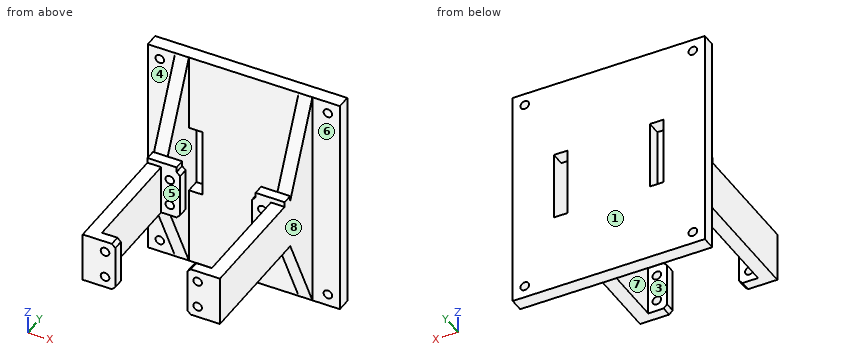
```python
from build123d import *

# Parameters (mm, degrees)
EXTRUDE_1_DEPTH      = 65
CUT_EXTRUDE_2_REACH  = 99.185
SKETCH_2_R           = 1.25
CUT_EXTRUDE_4_REACH  = 99.185
SKETCH_10_R          = 1.25
CUT_EXTRUDE_8_DEPTH  = 98.185389848
CUT_EXTRUDE_9_REACH  = 99.185
CUT_EXTRUDE_10_REACH = 99.185
SKETCH_25_W          = 8.5
SKETCH_25_H          = 3
EXTRUDE_2_DEPTH      = 1.5
SKETCH_26_W          = 8.5
SKETCH_26_H          = 3
EXTRUDE_3_DEPTH      = 1.5
CUT_EXTRUDE_11_REACH = 99.185


with BuildPart() as part:
    # 草图1 → 凸台-拉伸1 (new body)
    with BuildSketch(Plane.XY):
        Polygon((9.5, 3), (4, 3), (4, 35), (9.5, 35), (9.5, 38), (4, 38), (4, 50), (36, 50), (36, 38), (30.5, 38), (30.5, 35), (36, 35), (36, 3), (30.5, 3), (30.5, 0), (40, 0), (40, 50), (48, 50), (48, 54), (-8, 54), (-8, 50), (0, 50), (0, 0), (9.5, 0), align=None)
    extrude(amount=EXTRUDE_1_DEPTH)

    # 草图2 → 切除-拉伸2 (cut, up to next)
    with BuildSketch(Plane(origin=(0, 54, 0), x_dir=(1, 0, 0), z_dir=(0, 1, 0)), mode=Mode.PRIVATE) as cut_extrude_2_sk1:
        with Locations(Location((-4.5, -61.5, 0), (0, 0, 270))):
            Circle(SKETCH_2_R)
    cut_extrude_2_tool1 = extrude(cut_extrude_2_sk1.sketch, amount=-CUT_EXTRUDE_2_REACH, mode=Mode.PRIVATE) & part.part
    # 草图2 → 切除-拉伸2 (cut, up to next)
    with BuildSketch(Plane(origin=(0, 54, 0), x_dir=(1, 0, 0), z_dir=(0, 1, 0)), mode=Mode.PRIVATE) as cut_extrude_2_sk2:
        with Locations(Location((44.5, -61.5, 0), (0, 0, 270))):
            Circle(SKETCH_2_R)
    cut_extrude_2_tool2 = extrude(cut_extrude_2_sk2.sketch, amount=-CUT_EXTRUDE_2_REACH, mode=Mode.PRIVATE) & part.part
    # 草图2 → 切除-拉伸2 (cut, up to next)
    with BuildSketch(Plane(origin=(0, 54, 0), x_dir=(1, 0, 0), z_dir=(0, 1, 0)), mode=Mode.PRIVATE) as cut_extrude_2_sk3:
        with Locations(Location((44.5, -3.5, 0), (0, 0, 270))):
            Circle(SKETCH_2_R)
    cut_extrude_2_tool3 = extrude(cut_extrude_2_sk3.sketch, amount=-CUT_EXTRUDE_2_REACH, mode=Mode.PRIVATE) & part.part
    # 草图2 → 切除-拉伸2 (cut, up to next)
    with BuildSketch(Plane(origin=(0, 54, 0), x_dir=(1, 0, 0), z_dir=(0, 1, 0)), mode=Mode.PRIVATE) as cut_extrude_2_sk4:
        with Locations(Location((-4.5, -3.5, 0), (0, 0, 270))):
            Circle(SKETCH_2_R)
    cut_extrude_2_tool4 = extrude(cut_extrude_2_sk4.sketch, amount=-CUT_EXTRUDE_2_REACH, mode=Mode.PRIVATE) & part.part
    add(cut_extrude_2_tool1.solids().sort_by_distance((-4.5, 54, 61.5))[0], mode=Mode.SUBTRACT)
    add(cut_extrude_2_tool2.solids().sort_by_distance((44.5, 54, 61.5))[0], mode=Mode.SUBTRACT)
    add(cut_extrude_2_tool3.solids().sort_by_distance((44.5, 54, 3.5))[0], mode=Mode.SUBTRACT)
    add(cut_extrude_2_tool4.solids().sort_by_distance((-4.5, 54, 3.5))[0], mode=Mode.SUBTRACT)

    # 切除-拉伸4: up to this face of the body (flat: up to its plane)
    cut_extrude_4_end = Plane(part.part.faces().sort_by_distance((6.75, 38, 32.5))[0])
    # 草图10 → 切除-拉伸4 (cut, up to the picked face)
    with BuildSketch(Plane.XZ, mode=Mode.PRIVATE) as cut_extrude_4_sk1:
        with Locations((33.5, 36.5)):
            Circle(SKETCH_10_R)
    cut_extrude_4_tool1 = split(extrude(cut_extrude_4_sk1.sketch, amount=-CUT_EXTRUDE_4_REACH, mode=Mode.PRIVATE), bisect_by=cut_extrude_4_end, keep=Keep.BOTH, mode=Mode.PRIVATE)
    # 草图10 → 切除-拉伸4 (cut, up to the picked face)
    with BuildSketch(Plane.XZ, mode=Mode.PRIVATE) as cut_extrude_4_sk2:
        with Locations((33.5, 28.5)):
            Circle(SKETCH_10_R)
    cut_extrude_4_tool2 = split(extrude(cut_extrude_4_sk2.sketch, amount=-CUT_EXTRUDE_4_REACH, mode=Mode.PRIVATE), bisect_by=cut_extrude_4_end, keep=Keep.BOTH, mode=Mode.PRIVATE)
    # 草图10 → 切除-拉伸4 (cut, up to the picked face)
    with BuildSketch(Plane.XZ, mode=Mode.PRIVATE) as cut_extrude_4_sk3:
        with Locations(Location((6.5, 28.5, 0), (0, 0, 270))):
            Circle(SKETCH_10_R)
    cut_extrude_4_tool3 = split(extrude(cut_extrude_4_sk3.sketch, amount=-CUT_EXTRUDE_4_REACH, mode=Mode.PRIVATE), bisect_by=cut_extrude_4_end, keep=Keep.BOTH, mode=Mode.PRIVATE)
    # 草图10 → 切除-拉伸4 (cut, up to the picked face)
    with BuildSketch(Plane.XZ, mode=Mode.PRIVATE) as cut_extrude_4_sk4:
        with Locations(Location((6.5, 36.5, 0), (0, 0, 270))):
            Circle(SKETCH_10_R)
    cut_extrude_4_tool4 = split(extrude(cut_extrude_4_sk4.sketch, amount=-CUT_EXTRUDE_4_REACH, mode=Mode.PRIVATE), bisect_by=cut_extrude_4_end, keep=Keep.BOTH, mode=Mode.PRIVATE)
    add(cut_extrude_4_tool1.solids().sort_by(Axis((33.5, 0, 36.5), (0, 1, 0)))[0], mode=Mode.SUBTRACT)
    add(cut_extrude_4_tool2.solids().sort_by(Axis((33.5, 0, 28.5), (0, 1, 0)))[0], mode=Mode.SUBTRACT)
    add(cut_extrude_4_tool3.solids().sort_by(Axis((6.5, 0, 28.5), (0, 1, 0)))[0], mode=Mode.SUBTRACT)
    add(cut_extrude_4_tool4.solids().sort_by(Axis((6.5, 0, 36.5), (0, 1, 0)))[0], mode=Mode.SUBTRACT)

    # 草图20 → 切除-拉伸8 (cut, through all)
    with BuildSketch(Plane.ZY):
        Polygon((0, 50), (0, 0), (25.25, 0), (25.25, 38), align=None)
        Polygon((65, 50), (65, 0), (39.75, 0), (39.75, 38), align=None)
    extrude(amount=-CUT_EXTRUDE_8_DEPTH, mode=Mode.SUBTRACT)

    # 切除-拉伸9: up to this face of the body (flat: up to its plane)
    cut_extrude_9_end = Plane(part.part.faces().sort_by_distance((33.214903751, 38, 32.5))[0])
    # 草图21 → 切除-拉伸9 (cut, up to the picked face)
    with BuildSketch(Plane.XZ, mode=Mode.PRIVATE) as cut_extrude_9_sk1:
        Polygon((30.5, 38.75), (31.5, 39.75), (30.5, 39.75), align=None)
    cut_extrude_9_tool1 = split(extrude(cut_extrude_9_sk1.sketch, amount=-CUT_EXTRUDE_9_REACH, mode=Mode.PRIVATE), bisect_by=cut_extrude_9_end, keep=Keep.BOTH, mode=Mode.PRIVATE)
    # 草图21 → 切除-拉伸9 (cut, up to the picked face)
    with BuildSketch(Plane.XZ, mode=Mode.PRIVATE) as cut_extrude_9_sk2:
        Polygon((30.5, 26.25), (31.5, 25.25), (30.5, 25.25), align=None)
    cut_extrude_9_tool2 = split(extrude(cut_extrude_9_sk2.sketch, amount=-CUT_EXTRUDE_9_REACH, mode=Mode.PRIVATE), bisect_by=cut_extrude_9_end, keep=Keep.BOTH, mode=Mode.PRIVATE)
    add(cut_extrude_9_tool1.solids().sort_by(Axis((30.833333, 0, 39.416667), (0, 1, 0)))[0], mode=Mode.SUBTRACT)
    add(cut_extrude_9_tool2.solids().sort_by(Axis((30.833333, 0, 25.583333), (0, 1, 0)))[0], mode=Mode.SUBTRACT)

    # 切除-拉伸10: up to this face of the body (flat: up to its plane)
    cut_extrude_10_end = Plane(part.part.faces().sort_by_distance((6.785096249, 38, 32.5))[0])
    # 草图22 → 切除-拉伸10 (cut, up to the picked face)
    with BuildSketch(Plane(origin=(0, 0, 0), x_dir=(-1, 0, 0), z_dir=(0, -1, 0)), mode=Mode.PRIVATE) as cut_extrude_10_sk1:
        Polygon((-8.5, -39.75), (-9.5, -38.75), (-9.5, -39.75), align=None)
    cut_extrude_10_tool1 = split(extrude(cut_extrude_10_sk1.sketch, amount=-CUT_EXTRUDE_10_REACH, mode=Mode.PRIVATE), bisect_by=cut_extrude_10_end, keep=Keep.BOTH, mode=Mode.PRIVATE)
    # 草图22 → 切除-拉伸10 (cut, up to the picked face)
    with BuildSketch(Plane(origin=(0, 0, 0), x_dir=(-1, 0, 0), z_dir=(0, -1, 0)), mode=Mode.PRIVATE) as cut_extrude_10_sk2:
        Polygon((-9.5, -25.25), (-8.5, -25.25), (-9.5, -26.25), align=None)
    cut_extrude_10_tool2 = split(extrude(cut_extrude_10_sk2.sketch, amount=-CUT_EXTRUDE_10_REACH, mode=Mode.PRIVATE), bisect_by=cut_extrude_10_end, keep=Keep.BOTH, mode=Mode.PRIVATE)
    add(cut_extrude_10_tool1.solids().sort_by(Axis((9.166667, 0, 39.416667), (0, 1, 0)))[0], mode=Mode.SUBTRACT)
    add(cut_extrude_10_tool2.solids().sort_by(Axis((9.166667, 0, 25.583333), (0, 1, 0)))[0], mode=Mode.SUBTRACT)

    # 草图25 → 凸台-拉伸2 (add)
    with BuildSketch(Plane.XY.offset(39.75)):
        with Locations((4.25, 36.5)):
            Rectangle(SKETCH_25_W, SKETCH_25_H)
    extrude(amount=EXTRUDE_2_DEPTH)

    # 草图26 → 凸台-拉伸3 (add)
    with BuildSketch(Plane.XY.offset(39.75)):
        with Locations((35.75, 36.5)):
            Rectangle(SKETCH_26_W, SKETCH_26_H)
    extrude(amount=EXTRUDE_3_DEPTH)

    # 草图27 → 切除-拉伸11 (cut, up to next)
    with BuildSketch(Plane(origin=(0, 54, 0), x_dir=(1, 0, 0), z_dir=(0, 1, 0)), mode=Mode.PRIVATE) as cut_extrude_11_sk1:
        Polygon((4, -32.5), (4, -22.5), (8, -22.5), (8, -42.5), (4, -42.5), align=None)
    cut_extrude_11_tool1 = extrude(cut_extrude_11_sk1.sketch, amount=-CUT_EXTRUDE_11_REACH, mode=Mode.PRIVATE) & part.part
    # 草图27 → 切除-拉伸11 (cut, up to next)
    with BuildSketch(Plane(origin=(0, 54, 0), x_dir=(1, 0, 0), z_dir=(0, 1, 0)), mode=Mode.PRIVATE) as cut_extrude_11_sk2:
        Polygon((36, -32.5), (36, -22.5), (32, -22.5), (32, -42.5), (36, -42.5), align=None)
    cut_extrude_11_tool2 = extrude(cut_extrude_11_sk2.sketch, amount=-CUT_EXTRUDE_11_REACH, mode=Mode.PRIVATE) & part.part
    add(cut_extrude_11_tool1.solids().sort_by_distance((6, 54, 32.5))[0], mode=Mode.SUBTRACT)
    add(cut_extrude_11_tool2.solids().sort_by_distance((34, 54, 32.5))[0], mode=Mode.SUBTRACT)


solid = part.part
```
Verification items for the finished model (mm, model axes). Face numbers are marked on the shaded views. A direction names the side the tool comes from. Coordinates: 2 decimals unless noted, no trailing zeros. Loops run counter-clockwise (first coordinate to the right, second up) from the corner with the lowest first, then second, coordinate; pieces in that order, holes last. Notation, with made-up numbers: (45, 49.25) -> (77, 49.25) arc R10 cw to (77, 66.25) -> close; hole circle Ø3 at (41.5, 18.5). An arc over 180 degrees is marked (long way). Answer in a Markdown table with one row per item. Add a question column.
1. Section check A-A, the plane x = 6.5. Give the number of separate pieces and of enclosed holes in the cut face, then the cut area to 4 significant figures.
2. Section check B-B, the plane y = 26. Enter the section's corners in (x, z), then the cut area to 3 significant figures.
3. Depth check by flat-ended pin: P1, Ø16, axis at x = 19, z = 36.5, coming from the -Y side; P2, Ø10, axis at y = 19.5, z = 21, coming from the -X side; P3, Ø10, axis at x = 41, z = 47.5, coming from the -Y side. Enter the tip coordinate at first touch or a pass-through.
4. Access from +Z, -Z, +X, -X, +Y, -Y to the whole of each face (thin tool, end or side, straight path). Record for the marked faces 1, 2, 3 and 4.
5. Material ranges on probe 1 along Z at (x, y) = (33.5, 1.6); probe 2 along Y at (x, z) = (5, 35); probe 3 along Z at (x, y) = (33, 37), recorded low to high. Write a range as [from, to].
6. Draft check along Y on the marked faces 5, 6, 7 and 8. Enter one of: +Y half, -Y half, draft (parallel to the pull), parting line (faces both ways), or undercut.
7. Section check C-C, the plane z = 61.5. Enter the section's corners in (x, y).
Derived:
| question | item | result |
|---|---|---|
| 1 | separate pieces | 8 |
| 1 | enclosed holes | 0 |
| 1 | area | 241.5 mm² |
| 2 | outline | (0, 25.25) -> (4, 25.25) -> (4, 39.75) -> (0, 39.75) -> close; (36, 25.25) -> (40, 25.25) -> (40, 39.75) -> (36, 39.75) -> close |
| 2 | area | 116 mm² |
| 3 | P1 | stops at y = 50 |
| 3 | P2 | stops at x = 0 |
| 3 | P3 | stops at y = 39.35 |
| 4 | face 1 | +Z, -Z, +X, -X, +Y |
| 4 | face 2 | none |
| 4 | face 3 | +Z, -Z |
| 4 | face 4 | +Z, -Z, -X, -Y |
| 5 | probe 1 | z = [25.25, 27.25], [29.75, 35.25], [37.75, 39.75] |
| 5 | probe 2 | y = [0, 3], [35, 38] |
| 5 | probe 3 | z = [25.25, 27.35], [29.65, 35.35], [37.65, 41.25] |
| 6 | face 5 | undercut |
| 6 | face 6 | -Y half |
| 6 | face 7 | undercut |
| 6 | face 8 | draft |
| 7 | outline | (-8, 50) -> (-5.75, 50) -> (-5.75, 54) -> (-8, 54) -> close; (-3.25, 50) -> (0, 50) -> (0, 48.34) -> (4, 48.34) -> (4, 50) -> (36, 50) -> (36, 48.34) -> (40, 48.34) -> (40, 50) -> (43.25, 50) -> (43.25, 54) -> (-3.25, 54) -> close; (45.75, 50) -> (48, 50) -> (48, 54) -> (45.75, 54) -> close |
